Can you work these out from the model? Positions are in its coordinate system, mm. Face numbers are marked on the shaded views. A direction names the side the tool comes from. Give positions to 0.01 mm unless a question says otherwise; leave off trailing zeros. Order: outer loops, then holes, each group sorted by start corner. A loop starts at its lowest first (then second) coordinate and runs counter-clockwise, first axis right, second up.
Item 1: I want a section at C-C, the plane x = 44. Write out the boundary of the cut face in (y, z) (3 decimals), then the cut area to 3 significant figures.
Item 2: I want a section at D-D, the plane z = 2. Write out the boundary of the cut face in (x, y) (3 decimals), then the cut area to 3 significant figures.
Item 3: I'm going to push flat-ended pins straight in: pin 1 Ø4 at (x, y) = (6.35, 24.003) entering from +Z (3 decimals); pin 2 Ø7.5 at (x, z) = (28.5, 9) entering from +Y (3 decimals); pin 3 Ø2.5 at (x, z) = (52.832, 6.35) entering from -Y. Where does each tip first touch, or does it pass through?
Item 4: I want a section at A-A, the plane z = 6.35. Write out the boundary of the cut face in (x, y) (3 decimals).
Item 5: Which directions (+Z, -Z, +X, -X, +Y, -Y) give clear straight access to the entire face, cutting with the end or side of a thin tool? Please do the marked faces 1 and 2.
Item 6: I want a section at B-B, the plane x = 63.5. Write out the boundary of the cut face in (y, z) (3 decimals), then the cut area to 3 significant figures.
Item 7: If I drill on line 1 along Y through (x, z) = (6.35, 1.35); line 2 along Y through (x, z) = (25.5, 9.75) (3 decimals), over which ranges is the centre line in solid material (lowest first)?
```python
from build123d import *

# Parameters (mm, degrees)
F1_DEPTH = 69.85
F3_D     = 3.302
F5_D     = 3.302
F6_D     = 12.7


with BuildPart() as f1:
    # F0 (on Right) → F1 (new body)
    with BuildSketch(Plane.YZ):
        Polygon((0, 12.7), (0, 0), (44.45, 0), (44.45, 3.175), (3.175, 3.175), (3.175, 12.7), align=None)
    extrude(amount=F1_DEPTH)

    # F3 (through all)
    with Locations(Plane(origin=(0, 0, 0), x_dir=(1, 0, 0), z_dir=(0, 0, -1))):
        with Locations((6.35, -24.003), (63.5, -24.003)):
            Hole(F3_D / 2)

    # F5 (through all)
    with Locations(Plane.XZ):
        with Locations((52.832, 6.35)):
            Hole(F5_D / 2)

    # F6 (through all)
    with Locations(Plane(origin=(0, 0, 0), x_dir=(1, 0, 0), z_dir=(0, 0, -1))):
        with Locations((34.925, -16.002)):
            Hole(F6_D / 2)


solid = f1.part
```
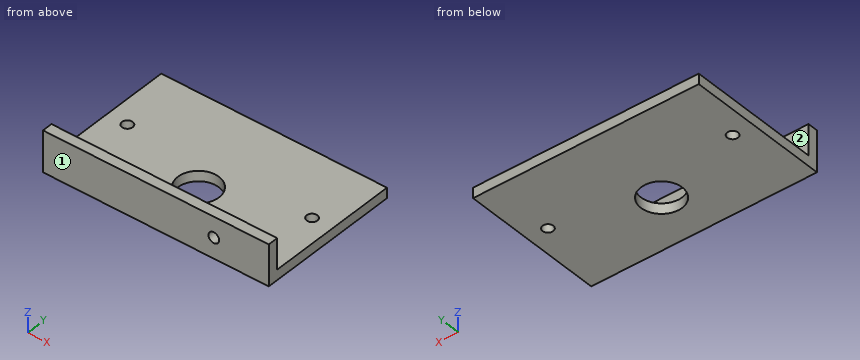
Results list:
1. outline: (0, 0) - (44.45, 0) - (44.45, 3.175) - (3.175, 3.175) - (3.175, 12.7) - (0, 12.7) - close
1. area: 171 mm2
2. outline: (0, 0) - (69.85, 0) - (69.85, 44.45) - (0, 44.45) - close; hole circle Ø3.302 at (6.35, 24.003); hole circle Ø12.7 at (34.925, 16.002); hole circle Ø3.302 at (63.5, 24.003)
2. area: 2,960 mm2
3. pin 1: stops at z = 3.175
3. pin 2: stops at y = 3.175
3. pin 3: passes through
4. outline: (0, 0) - (51.181, 0) - (51.181, 3.175) - (0, 3.175) - close; (54.483, 0) - (69.85, 0) - (69.85, 3.175) - (54.483, 3.175) - close
5. face 1: +Z, -Z, +X, -X, -Y
5. face 2: +Z, +X, -X, +Y
6. outline: (0, 0) - (22.352, 0) - (22.352, 3.175) - (3.175, 3.175) - (3.175, 12.7) - (0, 12.7) - close; (25.654, 0) - (44.45, 0) - (44.45, 3.175) - (25.654, 3.175) - close
6. area: 161 mm2
7. line 1: y = 0 to 22.35, 25.65 to 44.45
7. line 2: y = 0 to 3.175
